Part model, mm, in its own coordinate system. A direction names the side the tool comes from. Round coordinates to 2 decimals unless told otherwise and drop trailing zeros. Loops run counter-clockwise (first coordinate to the right, second up) from the corner with the lowest first, then second, coordinate; pieces in that order, holes last.
1) Probe line 1 (Y direction, x = -18.5, z = 14); line 2 (X direction, y = 12.5, z = 7.25); line 3 (Y direction, x = -22.55, z = 11.75). List the from-to ranges inside material, lowest first.
2) Mould opens along Y. For faces 1 (the flat face through (-6.596, 6, 14)), 2 (the flat face through (-28, 21.334, 4)), 3 (the flat face through (-38, 34, 7.5)) say: +Y half, -Y half, draft (parallel to the pull), parting line (faces both ways), or undercut.
3) Drop flat-ended pins along their axis: P1, Ø8, axis at x = -30, z = 3, coming from the +Y side; P2, Ø12, axis at y = 32, z = 11, coming from the +X side; P3, Ø4.5, axis at x = -14.5, y = 3.5, coming from the +Z side; P4, Ø14, axis at x = -33.5, y = 29.5, coming from the +Z side. Give the stop position or say it passes through.
4) 3-axis set-ups, long thin cutter, end or side, ignore diameter. For faces 4 (the cylindrical face through (-4.822, 6.106, 13.485)), 5 (the flat face through (-6.596, 30, 10)), 6 (the flat face through (-14, -10.166, 12)): which of +Z, -Z, +X, -X, +Y, -Y reach the whole face in a straight line?
5) Band-saw the part on B-B, the plane z = 11.75. State how many separate pieces and enclosed holes the cut face has, then the cut area to 3 significant figures.
6) Band-saw the part on C-C, the plane z = 16.25. Write the cut outline in (x, y).
7) Band-saw the part on A-A, the plane x = -12.5. Write the cut outline in (y, z).
8) Band-saw the part on D-D, the plane y = -2. Write the cut outline in (x, z).
from build123d import *

# Parameters (mm, degrees)
SKETCH1_W           = 22
SKETCH1_H           = 56
SKETCH1_W_2         = 15
SKETCH1_H_2         = 15
BOSS_EXTRUDE1_DEPTH = 20
SKETCH2_W           = 15
SKETCH2_H           = 15
SKETCH2_H_2         = 5.5
CUT_EXTRUDE1_DEPTH  = 15.5
SKETCH4_R           = 5.25
BOSS_EXTRUDE3_DEPTH = 7.5
FILLET4_R           = 1
SKETCH5_R           = 1.75
CUT_EXTRUDE2_DEPTH  = 10
CUT_EXTRUDE3_START  = -10
SKETCH6_R           = 1.75
CUT_EXTRUDE3_DEPTH  = 10


with BuildPart() as part:
    # Sketch1 → Boss-Extrude1 (new body)
    with BuildSketch(Plane.XY):
        with Locations((-14.096172604, 14.333947726)):
            Rectangle(SKETCH1_W, SKETCH1_H)
        with Locations((-14.096172604, 31.333947726)):
            Rectangle(SKETCH1_W_2, SKETCH1_H_2, mode=Mode.SUBTRACT)
    extrude(amount=BOSS_EXTRUDE1_DEPTH)

    # Sketch2 → Cut-Extrude1 (cut)
    with BuildSketch(Plane.XY.offset(20)):
        with Locations((-14.096172604, 6.333947726)):
            Rectangle(SKETCH2_W, SKETCH2_H)
        with Locations((-14.096172604, -7.416052274)):
            Rectangle(SKETCH2_W, SKETCH2_H_2)
    extrude(amount=-CUT_EXTRUDE1_DEPTH, mode=Mode.SUBTRACT)

    # Sketch4 → Boss-Extrude3 (add)
    with BuildSketch(Plane(origin=(0, 0, 0), x_dir=(-1, 0, 0), z_dir=(0, 0, -1))):
        with BuildLine():
            Line((32.596172604, 41.333947726), (25.096172604, 41.333947726))
            Line((25.096172604, 41.333947726), (25.096172604, 21.333947726))
            Line((25.096172604, 21.333947726), (32.596172604, 21.333947726))
            ThreePointArc((32.596172604, 21.333947726), (42.596172604, 31.333947726), (32.596172604, 41.333947726))
        make_face()
        with Locations((32.596172604, 31.333947726)):
            Circle(SKETCH4_R, mode=Mode.SUBTRACT)
    extrude(amount=-BOSS_EXTRUDE3_DEPTH)

    # Fillet4
    fillet4_edges = [part.edges().sort_by_distance(p)[0] for p in [
        (-3.096172604, 14.333947726, 20),
        (-14.096172604, 42.333947726, 20),
        (-25.096172604, 14.333947726, 20),
        (-14.096172604, 42.333947726, 0),
        (-3.096172604, 14.333947726, 0),
        (-25.096172604, 3.833947726, 0),
        (-25.096172604, 41.833947726, 0),
        (-25.096172604, 42.333947726, 10),
        (-3.096172604, 42.333947726, 10),
    ]]
    fillet(fillet4_edges, radius=FILLET4_R - 0.0001)  # a hair under: the kernel refuses the full size

    # Sketch5 → Cut-Extrude2 (cut)
    with BuildSketch(Plane(origin=(-3.096172604, 0, 0), x_dir=(0, 0, -1), z_dir=(1, 0, 0))):
        with Locations(Location((-11.75, 31.333947726, 0), (0, 0, 90))):
            Circle(SKETCH5_R)
        with Locations(Location((-11.75, 6.333947726, 0), (0, 0, 90))):
            Circle(SKETCH5_R)
    extrude(amount=-CUT_EXTRUDE2_DEPTH, mode=Mode.SUBTRACT)

    # Sketch6 → Cut-Extrude3 (cut)
    with BuildSketch(Plane.ZY.offset(25.096172604).offset(CUT_EXTRUDE3_START)):
        with Locations(Location((11.75, 6.333947726, 0), (0, 0, 90))):
            Circle(SKETCH6_R)
    extrude(amount=CUT_EXTRUDE3_DEPTH, mode=Mode.SUBTRACT)


solid = part.part
Reported:
1. line 1: y = -13.67 to -10.17, -4.67 to -1.17, 13.83 to 23.83, 38.83 to 42.33
1. line 2: x = -25.1 to -21.6, -6.6 to -3.1
1. line 3: y = -13.67 to 4.58, 8.08 to 42.33
2. face 1: undercut
2. face 2: -Y half
2. face 3: draft
3. P1: stops at y = 41.33
3. P2: stops at x = -3.1
3. P3: stops at z = 4.5
3. P4: stops at z = 7.5
4. face 4: +X, -X
4. face 5: +Z, -Z
4. face 6: +Z
5. separate pieces: 2
5. enclosed holes: 1
5. area: 662 mm2
6. outline: (-25.1, -13.67) - (-3.1, -13.67) - (-3.1, 41.33) arc R1 ccw to (-4.1, 42.33) - (-24.1, 42.33) arc R1 ccw to (-25.1, 41.33) - close; hole (-21.6, -10.17) - (-6.6, -10.17) - (-6.6, -4.67) - (-21.6, -4.67) - close; hole (-21.6, -1.17) - (-6.6, -1.17) - (-6.6, 13.83) - (-21.6, 13.83) - close; hole (-21.6, 23.83) - (-6.6, 23.83) - (-6.6, 38.83) - (-21.6, 38.83) - close
7. outline: (-13.67, 0) - (23.83, 0) - (23.83, 20) - (13.83, 20) - (13.83, 4.5) - (-1.17, 4.5) - (-1.17, 20) - (-4.67, 20) - (-4.67, 4.5) - (-10.17, 4.5) - (-10.17, 20) - (-13.67, 20) - close; (38.83, 0) - (41.33, 0) arc R1 ccw to (42.33, 1) - (42.33, 19) arc R1 ccw to (41.33, 20) - (38.83, 20) - close
8. outline: (-25.1, 1) arc R1 ccw to (-24.1, 0) - (-4.1, 0) arc R1 ccw to (-3.1, 1) - (-3.1, 19) arc R1 ccw to (-4.1, 20) - (-24.1, 20) arc R1 ccw to (-25.1, 19) - close
